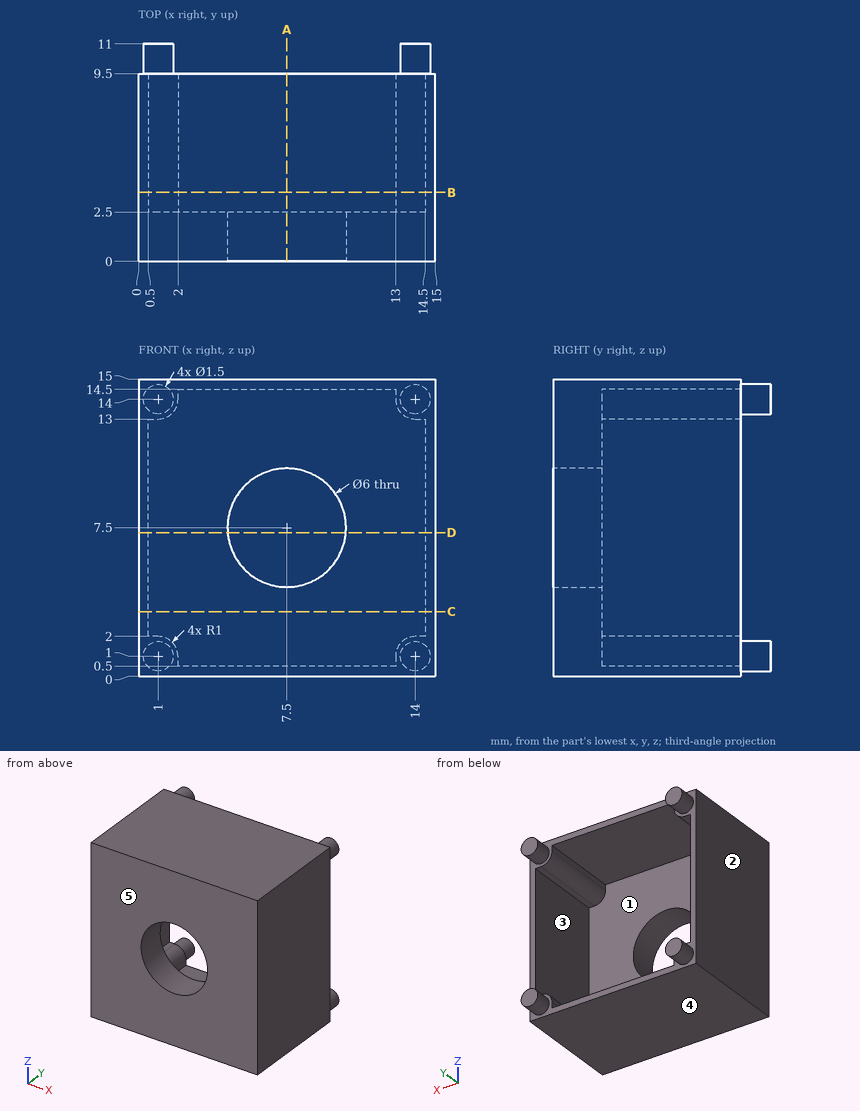
Geometry check sheet. Reference: drawing and pictorial views, mm from the part's lowest x, y, z. A direction names the side the tool comes from. Coordinates: 2 decimals unless noted, no trailing zeros. Order: outer loops, then holes, each group sorted by start corner. A loop starts at its lowest first (then second) coordinate and runs counter-clockwise, first axis right, second up.
Item 1: Section check D-D (z = 7.25). Enter the section's corners in (x, y), plus the area to 3 significant figures.
Item 2: Tool access check on the marked faces 1 and 2. Record the directions out of +Z, -Z, +X, -X, +Y, -Y that give a thin tool (end or side, any length) a straight path to the whole face; none if there is none.
Item 3: Scan lines: line 1 along X through (y, z) = (4.5, 4.5); line 2 along X through (y, z) = (1.1, 7.5). Record each from-to range of solid material in increasing order.
Item 4: Section check A-A (x = 7.5). Enter the section's corners in (y, z), plus the area to 3 significant figures.
Item 5: Mould release check, pull along Z, two halves, no side actions. Record for the marked faces 3, 4 and 5: released by +Z, released by -Z, zero draft, split by the parting line, or undercut.
Item 6: Section check B-B (y = 3.5). Enter the section's corners in (x, z).
Item 7: Depth check by flat-ended pin: pin 1 (5.5 mm diameter, centred on x = 7.5, z = 7.5, fed in from -Y); pin 2 (4.5 mm diameter, centred on x = 5.5, z = 9, fed in from +Y). Enter the tip coordinate at first touch or a pass-through.
Item 8: Section check C-C (z = 3.25). Enter the section's corners in (x, y).
Check sheet entries:
1. outline: (0, 0) - (4.51, 0) - (4.51, 2.5) - (0.5, 2.5) - (0.5, 9.5) - (0, 9.5) - close; (10.49, 0) - (15, 0) - (15, 9.5) - (14.5, 9.5) - (14.5, 2.5) - (10.49, 2.5) - close
1. area: 29.6 mm2
2. face 1: +Y
2. face 2: +Z, -Z, -X, +Y, -Y
3. line 1: x = 0 to 0.5, 14.5 to 15
3. line 2: x = 0 to 4.5, 10.5 to 15
4. outline: (0, 0) - (9.5, 0) - (9.5, 0.5) - (2.5, 0.5) - (2.5, 4.5) - (0, 4.5) - close; (0, 10.5) - (2.5, 10.5) - (2.5, 14.5) - (9.5, 14.5) - (9.5, 15) - (0, 15) - close
4. area: 29.5 mm2
5. face 3: undercut
5. face 4: released by -Z
5. face 5: zero draft
6. outline: (0, 0) - (15, 0) - (15, 15) - (0, 15) - close; hole (0.5, 2) - (1, 2) arc R1 cw to (2, 1) - (2, 0.5) - (13, 0.5) - (13, 1) arc R1 cw to (14, 2) - (14.5, 2) - (14.5, 13) - (14, 13) arc R1 cw to (13, 14) - (13, 14.5) - (2, 14.5) - (2, 14) arc R1 cw to (1, 13) - (0.5, 13) - close
7. pin 1: passes through
7. pin 2: stops at y = 2.5
8. outline: (0, 0) - (15, 0) - (15, 9.5) - (14.5, 9.5) - (14.5, 2.5) - (0.5, 2.5) - (0.5, 9.5) - (0, 9.5) - close
